from build123d import *

# Parameters (mm, degrees)
F1_DEPTH = 2.9718


with BuildPart() as f1:
    # F0 (on Right) → F1 (new body)
    with BuildSketch(Plane.YZ):
        with BuildLine():
            Line((76.2, -111.3282), (111.3282, -111.3282))
            Line((111.3282, -111.3282), (111.3282, -63.5))
            Line((111.3282, -63.5), (114.3, -63.5))
            Line((114.3, -63.5), (114.3, -45.6943407893))
            ThreePointArc((114.3, -45.6943407893), (111.252, -44.45), (114.3, -43.2056592107))
            Line((114.3, -43.2056592107), (114.3, -25.4))
            Line((114.3, -25.4), (111.3282, -25.4))
            Line((111.3282, -25.4), (111.3282, -1.7653))
            Line((111.3282, -1.7653), (101.1682, -1.7653))
            Line((101.1682, -1.7653), (101.1682, -3.8862))
            Line((101.1682, -3.8862), (98.5266, -3.8862))
            Line((98.5266, -3.8862), (98.5266, -1.7653))
            Line((98.5266, -1.7653), (93.4974, -1.7653))
            Line((93.4974, -1.7653), (93.4974, 1.7653))
            Line((93.4974, 1.7653), (98.5266, 1.7653))
            Line((98.5266, 1.7653), (98.5266, 3.8862))
            Line((98.5266, 3.8862), (101.1682, 3.8862))
            Line((101.1682, 3.8862), (101.1682, 1.7653))
            Line((101.1682, 1.7653), (111.3282, 1.7653))
            Line((111.3282, 1.7653), (111.3282, 25.4))
            Line((111.3282, 25.4), (114.3, 25.4))
            Line((114.3, 25.4), (114.3, 43.2056592107))
            ThreePointArc((114.3, 43.2056592107), (111.252, 44.45), (114.3, 45.6943407893))
            Line((114.3, 45.6943407893), (114.3, 63.5))
            Line((114.3, 63.5), (111.3282, 63.5))
            Line((111.3282, 63.5), (111.3282, 114.3))
            Line((111.3282, 114.3), (85.09, 114.3))
            Line((85.09, 114.3), (85.09, -69.85))
            Line((85.09, -69.85), (82.55, -69.85))
            Line((82.55, -69.85), (82.55, 114.3))
            Line((82.55, 114.3), (77.47, 114.3))
            Line((77.47, 114.3), (77.47, -69.85))
            Line((77.47, -69.85), (74.93, -69.85))
            Line((74.93, -69.85), (74.93, 114.3))
            Line((74.93, 114.3), (69.85, 114.3))
            Line((69.85, 114.3), (69.85, -69.85))
            Line((69.85, -69.85), (67.31, -69.85))
            Line((67.31, -69.85), (67.31, 114.3))
            Line((67.31, 114.3), (62.23, 114.3))
            Line((62.23, 114.3), (62.23, -69.85))
            Line((62.23, -69.85), (59.69, -69.85))
            Line((59.69, -69.85), (59.69, 114.3))
            Line((59.69, 114.3), (54.61, 114.3))
            Line((54.61, 114.3), (54.61, -69.85))
            Line((54.61, -69.85), (52.07, -69.85))
            Line((52.07, -69.85), (52.07, 114.3))
            Line((52.07, 114.3), (46.99, 114.3))
            Line((46.99, 114.3), (46.99, -69.85))
            Line((46.99, -69.85), (44.45, -69.85))
            Line((44.45, -69.85), (44.45, 114.3))
            Line((44.45, 114.3), (39.37, 114.3))
            Line((39.37, 114.3), (39.37, -69.85))
            Line((39.37, -69.85), (36.83, -69.85))
            Line((36.83, -69.85), (36.83, 114.3))
            Line((36.83, 114.3), (31.75, 114.3))
            Line((31.75, 114.3), (31.75, -69.85))
            Line((31.75, -69.85), (29.21, -69.85))
            Line((29.21, -69.85), (29.21, 114.3))
            Line((29.21, 114.3), (24.13, 114.3))
            Line((24.13, 114.3), (24.13, -69.85))
            Line((24.13, -69.85), (21.59, -69.85))
            Line((21.59, -69.85), (21.59, 114.3))
            Line((21.59, 114.3), (16.51, 114.3))
            Line((16.51, 114.3), (16.51, -69.85))
            Line((16.51, -69.85), (13.97, -69.85))
            Line((13.97, -69.85), (13.97, 114.3))
            Line((13.97, 114.3), (8.89, 114.3))
            Line((8.89, 114.3), (8.89, -69.85))
            Line((8.89, -69.85), (6.35, -69.85))
            Line((6.35, -69.85), (6.35, 114.3))
            Line((6.35, 114.3), (1.27, 114.3))
            Line((1.27, 114.3), (1.27, -69.85))
            Line((1.27, -69.85), (-1.27, -69.85))
            Line((-1.27, -69.85), (-1.27, 114.3))
            Line((-1.27, 114.3), (-6.35, 114.3))
            Line((-6.35, 114.3), (-6.35, -69.85))
            Line((-6.35, -69.85), (-8.89, -69.85))
            Line((-8.89, -69.85), (-8.89, 114.3))
            Line((-8.89, 114.3), (-13.97, 114.3))
            Line((-13.97, 114.3), (-13.97, -69.85))
            Line((-13.97, -69.85), (-16.51, -69.85))
            Line((-16.51, -69.85), (-16.51, 114.3))
            Line((-16.51, 114.3), (-21.59, 114.3))
            Line((-21.59, 114.3), (-21.59, -69.85))
            Line((-21.59, -69.85), (-24.13, -69.85))
            Line((-24.13, -69.85), (-24.13, 114.3))
            Line((-24.13, 114.3), (-29.21, 114.3))
            Line((-29.21, 114.3), (-29.21, -69.85))
            Line((-29.21, -69.85), (-31.75, -69.85))
            Line((-31.75, -69.85), (-31.75, 114.3))
            Line((-31.75, 114.3), (-36.83, 114.3))
            Line((-36.83, 114.3), (-36.83, -69.85))
            Line((-36.83, -69.85), (-39.37, -69.85))
            Line((-39.37, -69.85), (-39.37, 114.3))
            Line((-39.37, 114.3), (-44.45, 114.3))
            Line((-44.45, 114.3), (-44.45, -69.85))
            Line((-44.45, -69.85), (-46.99, -69.85))
            Line((-46.99, -69.85), (-46.99, 114.3))
            Line((-46.99, 114.3), (-52.07, 114.3))
            Line((-52.07, 114.3), (-52.07, -69.85))
            Line((-52.07, -69.85), (-54.61, -69.85))
            Line((-54.61, -69.85), (-54.61, 114.3))
            Line((-54.61, 114.3), (-59.69, 114.3))
            Line((-59.69, 114.3), (-59.69, -69.85))
            Line((-59.69, -69.85), (-62.23, -69.85))
            Line((-62.23, -69.85), (-62.23, 114.3))
            Line((-62.23, 114.3), (-67.31, 114.3))
            Line((-67.31, 114.3), (-67.31, -69.85))
            Line((-67.31, -69.85), (-69.85, -69.85))
            Line((-69.85, -69.85), (-69.85, 114.3))
            Line((-69.85, 114.3), (-74.93, 114.3))
            Line((-74.93, 114.3), (-74.93, -69.85))
            Line((-74.93, -69.85), (-77.47, -69.85))
            Line((-77.47, -69.85), (-77.47, 114.3))
            Line((-77.47, 114.3), (-82.55, 114.3))
            Line((-82.55, 114.3), (-82.55, -69.85))
            Line((-82.55, -69.85), (-85.09, -69.85))
            Line((-85.09, -69.85), (-85.09, 114.3))
            Line((-85.09, 114.3), (-111.3282, 114.3))
            Line((-111.3282, 114.3), (-111.3282, 63.5))
            Line((-111.3282, 63.5), (-114.3, 63.5))
            Line((-114.3, 63.5), (-114.3, 45.6943407893))
            ThreePointArc((-114.3, 45.6943407893), (-111.252, 44.45), (-114.3, 43.2056592107))
            Line((-114.3, 43.2056592107), (-114.3, 25.4))
            Line((-114.3, 25.4), (-111.3282, 25.4))
            Line((-111.3282, 25.4), (-111.3282, 1.7653))
            Line((-111.3282, 1.7653), (-101.1682, 1.7653))
            Line((-101.1682, 1.7653), (-101.1682, 3.8862))
            Line((-101.1682, 3.8862), (-98.5266, 3.8862))
            Line((-98.5266, 3.8862), (-98.5266, 1.7653))
            Line((-98.5266, 1.7653), (-93.4974, 1.7653))
            Line((-93.4974, 1.7653), (-93.4974, -1.7653))
            Line((-93.4974, -1.7653), (-98.5266, -1.7653))
            Line((-98.5266, -1.7653), (-98.5266, -3.8862))
            Line((-98.5266, -3.8862), (-101.1682, -3.8862))
            Line((-101.1682, -3.8862), (-101.1682, -1.7653))
            Line((-101.1682, -1.7653), (-111.3282, -1.7653))
            Line((-111.3282, -1.7653), (-111.3282, -25.4))
            Line((-111.3282, -25.4), (-114.3, -25.4))
            Line((-114.3, -25.4), (-114.3, -43.2056592107))
            ThreePointArc((-114.3, -43.2056592107), (-111.252, -44.45), (-114.3, -45.6943407893))
            Line((-114.3, -45.6943407893), (-114.3, -63.5))
            Line((-114.3, -63.5), (-111.3282, -63.5))
            Line((-111.3282, -63.5), (-111.3282, -111.3282))
            Line((-111.3282, -111.3282), (-76.2, -111.3282))
            Line((-76.2, -111.3282), (-76.2, -114.3))
            Line((-76.2, -114.3), (-64.7443407893, -114.3))
            ThreePointArc((-64.7443407893, -114.3), (-63.5, -111.252), (-62.2556592107, -114.3))
            Line((-62.2556592107, -114.3), (-50.8, -114.3))
            Line((-50.8, -114.3), (-50.8, -111.3282))
            Line((-50.8, -111.3282), (-33.5153, -111.3282))
            Line((-33.5153, -111.3282), (-33.5153, -101.1682))
            Line((-33.5153, -101.1682), (-35.6362, -101.1682))
            Line((-35.6362, -101.1682), (-35.6362, -98.5266))
            Line((-35.6362, -98.5266), (-33.5153, -98.5266))
            Line((-33.5153, -98.5266), (-33.5153, -93.4974))
            Line((-33.5153, -93.4974), (-29.9847, -93.4974))
            Line((-29.9847, -93.4974), (-29.9847, -98.5266))
            Line((-29.9847, -98.5266), (-27.8638, -98.5266))
            Line((-27.8638, -98.5266), (-27.8638, -101.1682))
            Line((-27.8638, -101.1682), (-29.9847, -101.1682))
            Line((-29.9847, -101.1682), (-29.9847, -111.3282))
            Line((-29.9847, -111.3282), (-12.7, -111.3282))
            Line((-12.7, -111.3282), (-12.7, -114.3))
            Line((-12.7, -114.3), (-1.2443407893, -114.3))
            ThreePointArc((-1.2443407893, -114.3), (0, -111.252), (1.2443407893, -114.3))
            Line((1.2443407893, -114.3), (12.7, -114.3))
            Line((12.7, -114.3), (12.7, -111.3282))
            Line((12.7, -111.3282), (29.9847, -111.3282))
            Line((29.9847, -111.3282), (29.9847, -101.1682))
            Line((29.9847, -101.1682), (27.8638, -101.1682))
            Line((27.8638, -101.1682), (27.8638, -98.5266))
            Line((27.8638, -98.5266), (29.9847, -98.5266))
            Line((29.9847, -98.5266), (29.9847, -93.4974))
            Line((29.9847, -93.4974), (33.5153, -93.4974))
            Line((33.5153, -93.4974), (33.5153, -98.5266))
            Line((33.5153, -98.5266), (35.6362, -98.5266))
            Line((35.6362, -98.5266), (35.6362, -101.1682))
            Line((35.6362, -101.1682), (33.5153, -101.1682))
            Line((33.5153, -101.1682), (33.5153, -111.3282))
            Line((33.5153, -111.3282), (50.8, -111.3282))
            Line((50.8, -111.3282), (50.8, -114.3))
            Line((50.8, -114.3), (62.2556592107, -114.3))
            ThreePointArc((62.2556592107, -114.3), (63.5, -111.252), (64.7443407893, -114.3))
            Line((64.7443407893, -114.3), (76.2, -114.3))
            Line((76.2, -114.3), (76.2, -111.3282))
        make_face()
    extrude(amount=F1_DEPTH)


solid = f1.part
Geometry check sheet. Reference: the model listing, model coordinates, mm. Give positions to 0.01 mm unless a question says otherwise; leave off trailing zeros.
1) Cross-section at A-A (z = -10.5). Count the separate pieces of the cut face and the enclosed holes in it, plus the area to 3 significant figures.
Values follow:
separate pieces: 24
enclosed holes: 0
area: 488 mm2
2) Thickness scan on line 1 (Z direction, x = 1.2, y = -113.03); line 2 (Y direction, x = 2.3, z = -113.03); line 3 (Z direction, x = 0.95, y = -104). Record the ranges inside material, lowest first.
Values follow:
line 1: z = -63.5 to -46.23, -42.67 to -25.4, 25.4 to 42.67, 46.23 to 63.5
line 2: y = -76.2 to -65.28, -61.72 to -50.8, -12.7 to -1.78, 1.78 to 12.7, 50.8 to 61.72, 65.28 to 76.2
line 3: z = -111.33 to -1.77, 1.77 to 114.3
3) Go/stop test with flat-tipped pins: pin 1 Ø0.6 at (x, y) = (1.5, -34.5) entering from -Z; pin 2 Ø2 at (y, z) = (113.03, 44.45) entering from +X; pin 3 Ø0.9 at (x, z) = (1.5, -10.5) entering from +Y; pin 4 Ø0.8 at (x, y) = (1.5, 15) entering from +Z. Record where each tip stops, or that it passes through.
Values follow:
pin 1: stops at z = -111.33
pin 2: passes through
pin 3: stops at y = 111.33
pin 4: stops at z = -69.85
